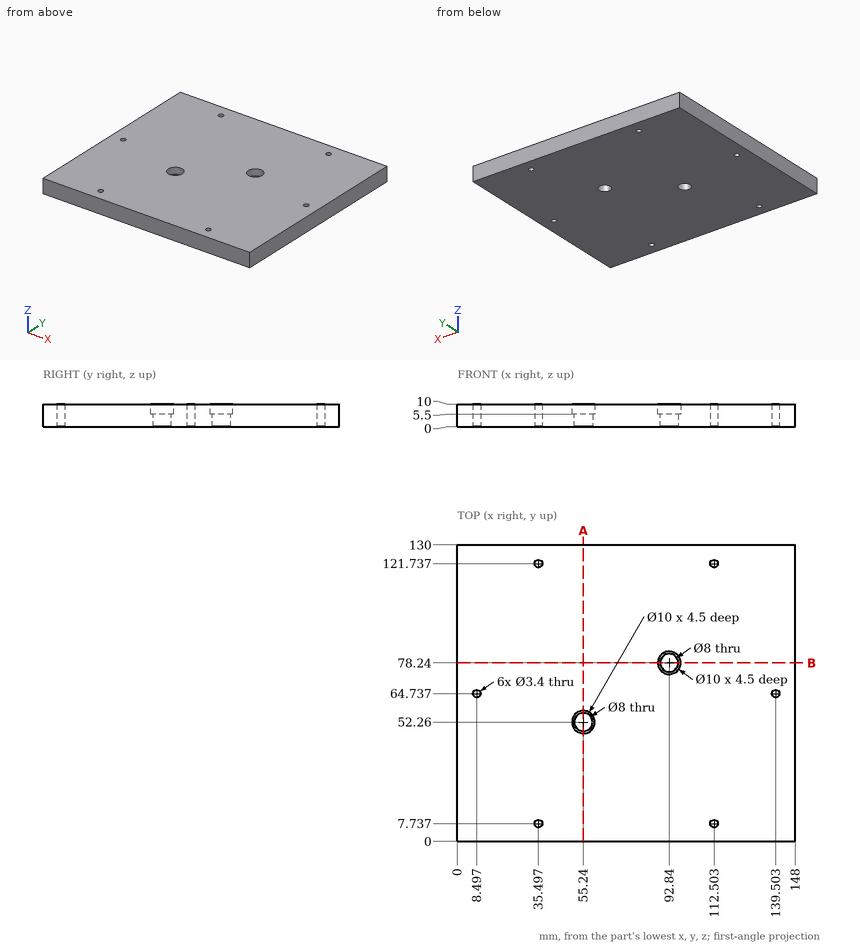
Study the drawing (mm; zero at the part's minimum x, y, z) and answer. Coordinates: 2 decimals unless noted, no trailing zeros. Loops run counter-clockwise (first coordinate to the right, second up) from the corner with the lowest first, then second, coordinate; pieces in that order, holes last. Notation, with made-up numbers: (60.25, 86) -> (100.25, 86) arc R31 cw to (100.25, 111) -> close; hole circle Ø11 at (40.5, 75.5). An arc over 180 degrees is marked (long way). Write item = value, one per line. Start each with the question number.
1) Given P1, Ø10.5, axis at x = 92.84, y = 78.24, coming from the -Z side; P2, Ø3, axis at x = 35.5, y = 121.74, coming from the -Z side; P3, Ø9, axis at x = 92.84, y = 78.24, coming from the +Z side, each flat-ended and moving along its own axis, determine where each tip first touches the part or whether it passes through.
2) Find the intervals of material crossed by L1, parallel to Y at x = 92.84, z = 8.55; L2, parallel to Y at x = 55.24, z = 7.65; L3, parallel to X at y = 79.5, z = 2, in increasing order. Write a range as from..to.
3) The part is cut by section A-A, the plane x = 55.24. Determine the outline of the cut face in (y, z), plus the area to 3 significant figures.
4) The part is cut by section B-B, the plane y = 78.24. Determine the outline of the cut face in (x, z), plus the area to 3 significant figures.
Result:
q1.P1 = 0
q1.P2 = through
q1.P3 = 5.5
q2.L1 = 0..73.24, 83.24..130
q2.L2 = 0..47.26, 57.26..130
q2.L3 = 0..89.04, 96.64..148
q3.outline = (0, 0) -> (48.26, 0) -> (48.26, 5.5) -> (47.26, 5.5) -> (47.26, 10) -> (0, 10) -> close; (56.26, 0) -> (130, 0) -> (130, 10) -> (57.26, 10) -> (57.26, 5.5) -> (56.26, 5.5) -> close
q3.area = 1,210 mm²
q4.outline = (0, 0) -> (88.84, 0) -> (88.84, 5.5) -> (87.84, 5.5) -> (87.84, 10) -> (0, 10) -> close; (96.84, 0) -> (148, 0) -> (148, 10) -> (97.84, 10) -> (97.84, 5.5) -> (96.84, 5.5) -> close
q4.area = 1,390 mm²
